Check sheet for the modelled part. Datum: model origin and axes. Units: mm. A direction names the side the tool comes from. Give positions to 0.01 mm unless a question says otherwise; leave off trailing zeros. Loops run counter-clockwise (first coordinate to the right, second up) from the corner with the lowest first, then second, coordinate; pieces in that order, holes last.
```python
from build123d import *

# Parameters (mm, degrees)
SKETCH1_W           = 73.025
SKETCH1_H           = 79.375
BOSS_EXTRUDE1_DEPTH = 63.5
SKETCH2_R           = 15.875
BOSS_EXTRUDE2_DEPTH = 12.7
SKETCH3_R           = 30.1625
BOSS_EXTRUDE3_DEPTH = 3.175
SKETCH4_R           = 17.4625
BOSS_EXTRUDE4_DEPTH = 6.35
SKETCH5_R           = 19.05
BOSS_EXTRUDE5_DEPTH = 6.35
FILLET1_R           = 2.54
FILLET2_R           = 2.54
FILLET5_R           = 2.54
SKETCH7_R           = 12.7
BOSS_EXTRUDE7_DEPTH = 25.4
FILLET6_R           = 6.35
SKETCH8_R           = 3.086351458
BOSS_EXTRUDE8_DEPTH = 38.1


with BuildPart() as part:
    # Sketch1 → Boss-Extrude1 (new body)
    with BuildSketch(Plane(origin=(0, 0, 0), x_dir=(1, 0, 0), z_dir=(0, 1, 0))):
        with Locations((36.5125, 39.6875)):
            Rectangle(SKETCH1_W, SKETCH1_H)
    extrude(amount=BOSS_EXTRUDE1_DEPTH)

    # Sketch2 → Boss-Extrude2 (add)
    with BuildSketch(Plane(origin=(0, 63.5, 0), x_dir=(1, 0, 0), z_dir=(0, 1, 0))):
        with Locations(Location((36.5125, 39.6875, 0), (0, 0, 270))):
            Circle(SKETCH2_R)
    extrude(amount=BOSS_EXTRUDE2_DEPTH)

    # Sketch3 → Boss-Extrude3 (add)
    with BuildSketch(Plane(origin=(0, 63.5, 0), x_dir=(1, 0, 0), z_dir=(0, 1, 0))):
        with Locations(Location((36.5125, 39.6875, 0), (0, 0, 90))):
            Circle(SKETCH3_R)
    extrude(amount=BOSS_EXTRUDE3_DEPTH)

    # Sketch4 → Boss-Extrude4 (add)
    with BuildSketch(Plane(origin=(0, 76.2, 0), x_dir=(1, 0, 0), z_dir=(0, 1, 0))):
        with Locations(Location((36.5125, 39.6875, 0), (0, 0, 270))):
            Circle(SKETCH4_R)
    extrude(amount=BOSS_EXTRUDE4_DEPTH)

    # Sketch5 → Boss-Extrude5 (add)
    with BuildSketch(Plane(origin=(0, 82.55, 0), x_dir=(1, 0, 0), z_dir=(0, 1, 0))):
        with Locations(Location((36.5125, 39.6875, 0), (0, 0, 270))):
            Circle(SKETCH5_R)
    extrude(amount=BOSS_EXTRUDE5_DEPTH)

    # Fillet1
    # the kernel refuses this fillet: 2.54 mm, written as the material it takes off along each edge
    with BuildSketch(Plane(origin=(36.5125, 82.55, -39.6875), x_dir=(0, 0, 1), z_dir=(-1, 0, 0))) as fillet1_piece_1:
        with BuildLine():
            CenterArc((16.51, 2.35464302), FILLET1_R, 292.024312837, 67.975687163)
            Line((17.4625, 0), (17.48155, -0.04709286))
            ThreePointArc((17.48155, -0.04709286), (18.25625, -0.0508), (19.05, -0.0508))
            Line((19.05, -0.0508), (19.1008, 0))
            Line((19.1008, 0), (19.1008, 2.35464302))
            Line((19.1008, 2.35464302), (19.05, 2.35464302))
        make_face()
    revolve(axis=Axis((36.5125, 82.55, -39.6875), (0, 1, 0)), mode=Mode.SUBTRACT)
    with BuildSketch(Plane(origin=(36.5125, 88.9, -39.6875), x_dir=(0, 0, 1), z_dir=(-1, 0, 0))) as fillet1_piece_2:
        with BuildLine():
            CenterArc((19.05 - FILLET1_R, -FILLET1_R), FILLET1_R, 0, 90)
            Line((19.05 - FILLET1_R, 0), (19.05 - FILLET1_R, FILLET1_R * 0.02))
            Line((19.05 - FILLET1_R, FILLET1_R * 0.02), (19.05 + FILLET1_R * 0.02, FILLET1_R * 0.02))
            Line((19.05 + FILLET1_R * 0.02, FILLET1_R * 0.02), (19.05 + FILLET1_R * 0.02, -FILLET1_R))
            Line((19.05 + FILLET1_R * 0.02, -FILLET1_R), (19.05, -FILLET1_R))
        make_face()
    revolve(axis=Axis((36.5125, 88.9, -39.6875), (0, 1, 0)), mode=Mode.SUBTRACT)

    # Fillet2
    fillet2_edges = [part.edges().sort_by_distance(p)[0] for p in [
        (0, 31.75, 0),
        (73.025, 31.75, 0),
        (73.025, 31.75, -79.375),
        (0, 31.75, -79.375),
    ]]
    fillet(fillet2_edges, radius=FILLET2_R)

    # Fillet5
    fillet5_edges = [part.edges().sort_by_distance(p)[0] for p in [
        (36.5125, 63.5, -79.375),
        (73.025, 63.5, -39.6875),
        (0, 63.5, -39.6875),
        (36.5125, 63.5, 0),
        (0.743948776, 63.5, -78.631051224),
        (0.743948776, 63.5, -0.743948776),
        (72.281051224, 63.5, -0.743948776),
        (72.281051224, 63.5, -78.631051224),
    ]]
    fillet(fillet5_edges, radius=FILLET5_R)

    # Sketch7 → Boss-Extrude7 (add)
    with BuildSketch(Plane.XY):
        with Locations(Location((36.5125, 14.834220105, 0), (0, 0, 180))):
            Circle(SKETCH7_R)
    extrude(amount=BOSS_EXTRUDE7_DEPTH)

    # Fillet6
    fillet6_edges = [part.edges().sort_by_distance(p)[0] for p in [
        (49.2125, 14.834220105, 25.4),
    ]]
    fillet(fillet6_edges, radius=FILLET6_R)

    # Sketch8 → Boss-Extrude8 (add)
    with BuildSketch(Plane.XY.offset(25.4)):
        with Locations(Location((38.506076801, 17.440379035, 0), (0, 0, 61.105176003))):
            Circle(SKETCH8_R)
        with Locations(Location((34.596139796, 12.429051324, 0), (0, 0, 180))):
            Circle(SKETCH8_R)
    extrude(amount=BOSS_EXTRUDE8_DEPTH)


solid = part.part
```
(1) Gauge pin test, flat ends, axial feed: pin 1 Ø5 at (x, y) = (48, 79.5) entering from -Z; pin 2 Ø10 at (x, y) = (28.5, 66.5) entering from +Z; pin 3 Ø18.5 at (x, y) = (23, 33) entering from +Z. Record the tip position at first contact, or that the pin passes through.
(2) Material ranges on line 1 (Y direction, x = 56.5, z = -68); line 2 (Y direction, x = 41, z = -59.5) (3 decimals); line 3 (Z direction, x = 68, y = 21) (3 decimals), recorded low to high.
(3) Section check B-B on y = 56. Record the boundary of the cut face in (x, z) (3 decimals).
(4) Section check D-D on z = 29. Record the boundary of the cut face in (x, y).
(5) Section check A-A on z = -6. Record the boundary of the cut face in (x, y) (3 decimals).
(6) Release check for a two-part mould opening along Y. For faces 4 (the face through (49.2, 14.3, 9.4)), 5 (the face through (40.919, 19.365, 44.183)), 6 (the face through (36, 30, -79.375)) record: pulls with the +Y half, pulls with the -Y half, needs draft (parallel to the pull), parting line crosses it, or undercut.
(7) Section check C-C on x = 61.5. Record the boundary of the cut face in (y, z) (3 decimals), plus the area to 3 significant figures.
(8) Access from +Z, -Z, +X, -X, +Y, -Y to the whole of each face (thin tool, end or side, straight path). Record for faces 1 (the face through (32.937, 9.827, 44.183)), 2 (the face through (37.21, 71.371, -55.547)), 3 (the face through (6, 63.5, -40)).
Computed values:
1. pin 1: stops at z = -54.66
1. pin 2: stops at z = -0.06
1. pin 3: stops at z = 0
2. line 1: y = 0 to 63.5
2. line 2: y = 0 to 66.675
2. line 3: z = -79.375 to 0
3. outline: (0, -76.835) arc R2.54 ccw to (2.54, -79.375) - (70.485, -79.375) arc R2.54 ccw to (73.025, -76.835) - (73.025, -2.54) arc R2.54 ccw to (70.485, 0) - (2.54, 0) arc R2.54 ccw to (0, -2.54) - close
4. outline: circle Ø6.17 at (34.6, 12.43); circle Ø6.17 at (38.51, 17.44)
5. outline: (0, 0) - (73.025, 0) - (73.025, 60.96) arc R2.54 ccw to (70.485, 63.5) - (2.54, 63.5) arc R2.54 ccw to (0, 60.96) - close
6. face 4: parting line crosses it
6. face 5: undercut
6. face 6: needs draft
7. outline: (0, -79.375) - (60.96, -79.375) arc R2.54 ccw to (63.5, -76.835) - (63.5, -56.581) - (66.675, -56.581) - (66.675, -22.794) - (63.5, -22.794) - (63.5, -2.54) arc R2.54 ccw to (60.96, 0) - (0, 0) - close
7. area: 5,140 mm2
8. face 1: +Z
8. face 2: none
8. face 3: +Y
